Source: three-view drawing plus pictorial views. Frame: mm from the lowest corner of the part. A direction names the side the tool comes from. Coordinates: 2 decimals unless noted, no trailing zeros. Write each loop counter-clockwise with the first axis right and the second up, starting at its lowest first coordinate (ties: lowest second). Pieces come first, ordered by that corner, then holes.
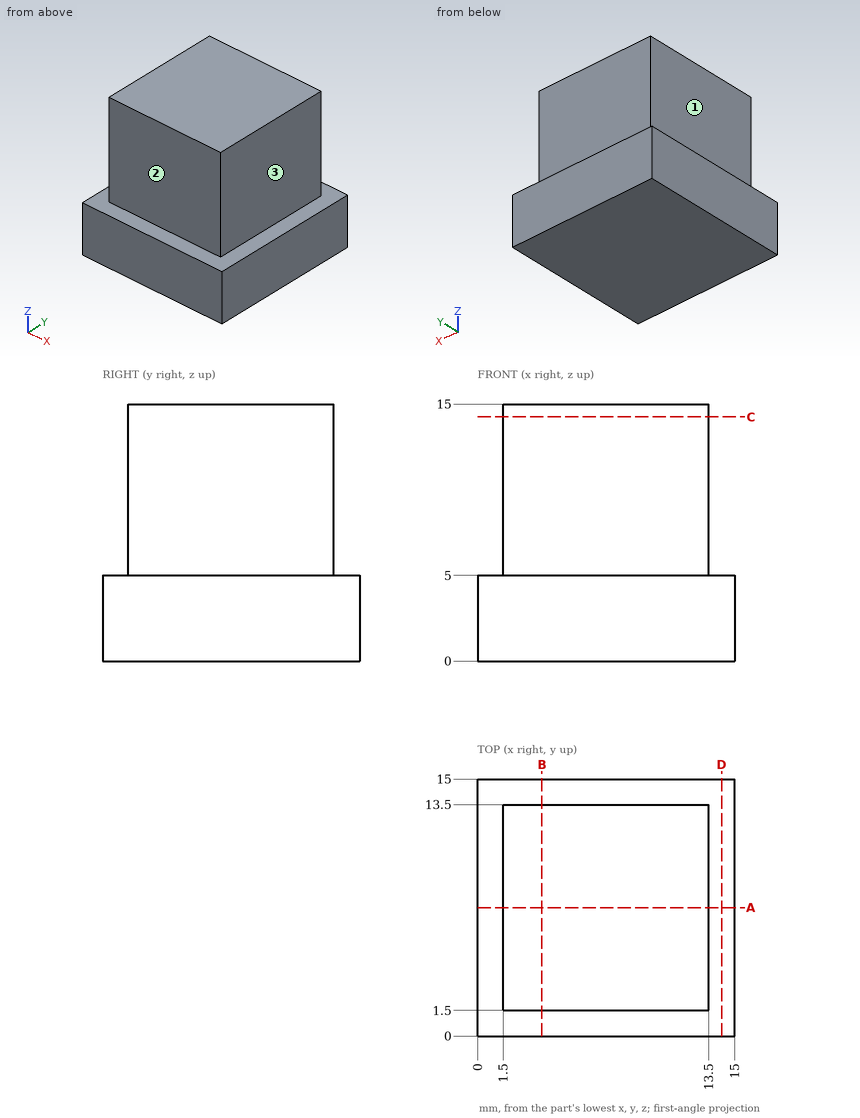
Item 1: Section query A-A, the plane y = 7.5. Return loops of the section in (x, z), then the cut area to 3 significant figures.
Item 2: Access query for the marked faces 1, 2 and 3. Directions: +Z, -Z, +X, -X, +Y, -Y. A direction counts if a zero-diameter tool reaches every point of the face in a straight line with its end or side. Return the directions, or none.
Item 3: Material intervals for line 1 (Y direction, x = 2.5, z = 10.5); line 2 (Z direction, x = 11, y = 1.25), sorted ascending.
Item 4: Pin query (flat end, axial travel): pin 1 Ø1.5 at (x, z) = (10.5, 8.5) entering from +Y; pin 2 Ø5 at (x, z) = (5, 10) entering from -Y. Return the tip coordinate at first contact, or that it passes through.
Item 5: Section query D-D, the plane x = 14.25. Return loops of the section in (y, z).
Item 6: Section query C-C, the plane z = 14.25. Return loops of the section in (x, y).
The answers:
1. outline: (0, 0) - (15, 0) - (15, 5) - (13.5, 5) - (13.5, 15) - (1.5, 15) - (1.5, 5) - (0, 5) - close
1. area: 195 mm2
2. face 1: +Z, -X, +Y, -Y
2. face 2: +Z, +X, -X, -Y
2. face 3: +Z, +X, +Y, -Y
3. line 1: y = 1.5 to 13.5
3. line 2: z = 0 to 5
4. pin 1: stops at y = 13.5
4. pin 2: stops at y = 1.5
5. outline: (0, 0) - (15, 0) - (15, 5) - (0, 5) - close
6. outline: (1.5, 1.5) - (13.5, 1.5) - (13.5, 13.5) - (1.5, 13.5) - close
